Geometry: final body of the model. Coordinates: model frame, mm. A direction names the side the tool comes from. Give positions to 0.01 mm unless a question says otherwise; leave off trailing zeros. Write each loop counter-clockwise with the first axis right and the second up, starting at its lowest first coordinate (ties: lowest second). Pieces come first, ordered by that corner, then holes.
```python
from build123d import *

# Parameters (mm, degrees)
PAD001_DEPTH    = 3
SKETCH010_R     = 2
POCKET007_DEPTH = 3.001
SKETCH011_R     = 2.5
POCKET008_DEPTH = 3.001


with BuildPart() as part:
    # Sketch004 → Pad001 (new body)
    with BuildSketch(Plane.YZ):
        Polygon((-35, 38), (-20, 38), (-20, 35), (20, 35), (20, 38), (35, 38), (35, 0), (15, 0), (15, -5), (10, -5), (10, -8), (-10, -8), (-10, -5), (-15, -5), (-15, 0), (-35, 0), align=None)
    extrude(amount=PAD001_DEPTH)

    # Sketch010 → Pocket007 (cut, through all)
    with BuildSketch(Plane.YZ.offset(3)):
        with Locations((-13, 29)):
            Circle(SKETCH010_R)
        with Locations((13, 29)):
            Circle(SKETCH010_R)
        with Locations((-13, 7)):
            Circle(SKETCH010_R)
        with Locations((13, 7)):
            Circle(SKETCH010_R)
        with BuildLine():
            Line((-20, 25), (-20, 12))
            ThreePointArc((-20, 12), (-17.5, 9.5), (-15, 12))
            Line((-15, 25), (-15, 12))
            ThreePointArc((-15, 25), (-17.5, 27.5), (-20, 25))
        make_face()
    extrude(amount=-POCKET007_DEPTH, mode=Mode.SUBTRACT)

    # Sketch011 → Pocket008 (cut, through all)
    with BuildSketch(Plane.YZ.offset(3)):
        with Locations((-27.5, 26)):
            Circle(SKETCH011_R)
        with Locations((27.5, 26)):
            Circle(SKETCH011_R)
    extrude(amount=-POCKET008_DEPTH, mode=Mode.SUBTRACT)


solid = part.part
```
Item 1: Section A-A, the plane y = -17.5. Return the cut outline in (x, z), plus the area to 3 significant figures.
Found:
outline: (0, 0) - (3, 0) - (3, 9.5) - (0, 9.5) - close; (0, 27.5) - (3, 27.5) - (3, 35) - (0, 35) - close
area: 51.0 mm2
Item 2: Pin query (flat end, axial travel): pin 1 Ø1 at (x, y) = (0.5, -11.5) entering from -Z; pin 2 Ø0.9 at (x, y) = (1.5, 25) entering from -Z; pin 3 Ø0.9 at (x, z) = (1.5, -3) entering from +Y. Return the tip coordinate at first contact, or that it passes through.
Found:
pin 1: stops at z = -5
pin 2: stops at z = 0
pin 3: stops at y = 15
Item 3: Pull-direction query (Y, two-part tool) for faces 1 (the face through (1, 0, -8)), 2 (the face through (1, 10, -6)), 3 (the face through (2, -20, 19)); classes: +Y half, -Y half, draft (parallel to the pull), parting line (faces both ways), or undercut.
Found:
face 1: draft
face 2: +Y half
face 3: undercut
Item 4: Section C-C, the plane y = 29. Return the cut outline in (x, z).
Found:
outline: (0, 0) - (3, 0) - (3, 24) - (0, 24) - close; (0, 28) - (3, 28) - (3, 38) - (0, 38) - close
Item 5: Reachability of faces 4 (the face through (2, -15, 19)), 5 (the face through (1, -20, 37)), 6 (the face through (1, 13, -5)), 7 (the face through (1, -12, -5)) from +Z, -Z, +X, -X, +Y, -Y: full face, straight path, thin tool, end or side. Return the list, or none.
Found:
face 4: +X, -X
face 5: +Z, +X, -X
face 6: -Z, +X, -X, +Y
face 7: -Z, +X, -X, -Y
Item 6: Section B-B, the plane x = 0.95. Return the cut outline in (y, z).
Found:
outline: (-35, 0) - (-15, 0) - (-15, -5) - (-10, -5) - (-10, -8) - (10, -8) - (10, -5) - (15, -5) - (15, 0) - (35, 0) - (35, 38) - (20, 38) - (20, 35) - (-20, 35) - (-20, 38) - (-35, 38) - close; hole circle Ø5 at (-27.5, 26); hole (-20, 12) arc R2.5 ccw to (-15, 12) - (-15, 25) arc R2.5 ccw to (-20, 25) - close; hole circle Ø4 at (-13, 7); hole circle Ø4 at (-13, 29); hole circle Ø4 at (13, 7); hole circle Ø4 at (13, 29); hole circle Ø5 at (27.5, 26)
Item 7: Line query: L1, parallel to Z at x = 1, y = 13; L2, parallel to Y at x = 1.1, z = 14; L3, parallel to Z at x = 1.7, y = -27.5. Output: solid intervals per line, ascending.
Found:
L1: z = -5 to 5, 9 to 27, 31 to 35
L2: y = -35 to -20, -15 to 35
L3: z = 0 to 23.5, 28.5 to 38
